```python
from build123d import *

# Parameters (mm, degrees)
SKETCH1_W               = 1.5
SKETCH1_H               = 620
BOSS_EXTRUDE1_DEPTH     = 1.5
BOSS_EXTRUDE3_DEPTH     = 1.5
SKETCH5_W               = 1.5
SKETCH5_H               = 1.5
CUT_EXTRUDE1_DEPTH      = 1
CUT_EXTRUDE1_DEPTH_BACK = 621
BOSS_EXTRUDE4_DEPTH     = 620
SKETCH6_R               = 5
CUT_EXTRUDE2_DEPTH      = 1
CUT_EXTRUDE2_DEPTH_BACK = 57.5
SKETCH7_R               = 5
CUT_EXTRUDE3_DEPTH      = 1
CUT_EXTRUDE3_DEPTH_BACK = 57.5


with BuildPart() as part:
    # Sketch1 → Boss-Extrude1 (new body)
    with BuildSketch(Plane(origin=(0, 0, 0), x_dir=(0, 0, -1), z_dir=(1, 0, 0))):
        Polygon((0, 255), (0, -255), (55, -310), (55, 310), align=None)
        with Locations((55.75, 0)):
            Rectangle(SKETCH1_W, SKETCH1_H)
    extrude(amount=BOSS_EXTRUDE1_DEPTH)

    # Sketch2 → Boss-Extrude3 (add)
    with BuildSketch(Plane(origin=(0, 0, -56.5), x_dir=(-1, 0, 0), z_dir=(0, 0, -1))):
        Polygon((55, 255), (55, -255), (0, -310), (0, 310), align=None)
    extrude(amount=-BOSS_EXTRUDE3_DEPTH)

    # Sketch5 → Cut-Extrude1 (cut, two sides)
    with BuildSketch(Plane.XZ.offset(310)) as cut_extrude1_sk:
        with BuildLine():
            ThreePointArc((1.5, -44.5), (-2.014718626, -52.985281374), (-10.5, -56.5))
            Line((-10.5, -56.5), (0, -56.5))
            Line((0, -56.5), (0, -55))
            Line((0, -55), (1.5, -55))
            Line((1.5, -55), (1.5, -44.5))
        make_face()
        with Locations((0.75, -55.75)):
            Rectangle(SKETCH5_W, SKETCH5_H)
    extrude(amount=CUT_EXTRUDE1_DEPTH, mode=Mode.SUBTRACT)
    extrude(cut_extrude1_sk.sketch, amount=-CUT_EXTRUDE1_DEPTH_BACK, mode=Mode.SUBTRACT)

    # Sketch5<3> → Boss-Extrude4 (add)
    with BuildSketch(Plane.XZ.offset(310)):
        with BuildLine():
            Line((-10.5, -55), (-10.5, -56.5))
            ThreePointArc((-10.5, -56.5), (-2.014718626, -52.985281374), (1.5, -44.5))
            Line((1.5, -44.5), (0, -44.5))
            ThreePointArc((0, -44.5), (-3.075378798, -51.924621202), (-10.5, -55))
        make_face()
    extrude(amount=-BOSS_EXTRUDE4_DEPTH)

    # Sketch6 → Cut-Extrude2 (cut, two sides)
    with BuildSketch(Plane(origin=(1.5, 0, 0), x_dir=(0, 0, -1), z_dir=(1, 0, 0))) as cut_extrude2_sk:
        with Locations((24.5, 0)):
            Circle(SKETCH6_R)
    extrude(amount=CUT_EXTRUDE2_DEPTH, mode=Mode.SUBTRACT)
    extrude(cut_extrude2_sk.sketch, amount=-CUT_EXTRUDE2_DEPTH_BACK, mode=Mode.SUBTRACT)

    # Sketch7 → Cut-Extrude3 (cut, two sides)
    with BuildSketch(Plane(origin=(0, 0, -56.5), x_dir=(-1, 0, 0), z_dir=(0, 0, -1))) as cut_extrude3_sk:
        with Locations((30.5, 0)):
            Circle(SKETCH7_R)
    extrude(amount=CUT_EXTRUDE3_DEPTH, mode=Mode.SUBTRACT)
    extrude(cut_extrude3_sk.sketch, amount=-CUT_EXTRUDE3_DEPTH_BACK, mode=Mode.SUBTRACT)


solid = part.part
```
Geometry check sheet. Reference: the model listing, model coordinates, mm. A direction names the side the tool comes from. Give positions to 0.01 mm unless a question says otherwise; leave off trailing zeros. Order: outer loops, then holes, each group sorted by start corner. A loop starts at its lowest first (then second) coordinate and runs counter-clockwise, first axis right, second up.
1. Thickness scan on L1, parallel to Y at x = 0.95, z = -24.5; L2, parallel to X at y = 90.5, z = -23; L3, parallel to Z at x = -31.5, y = 165. Record the ranges inside material, lowest first.
2. Section check C-C, the plane z = -13. Enter the section's corners in (x, y), and give its area (3 significant figures).
3. Section check A-A, the plane y = -206.5. Enter the section's corners in (x, z), and give its area (3 significant figures).
4. Release check for a two-part mould opening along Y. For faces 1 (the face through (0.76, 0.22, -19.505)), 2 (the face through (1, -277, -22)), 3 (the face through (-38, 4, -55)) record: pulls with the +Y half, pulls with the -Y half, needs draft (parallel to the pull), parting line crosses it, or undercut.
5. Access from +Z, -Z, +X, -X, +Y, -Y to the whole of each face (thin tool, end or side, straight path). Record for faces 4 (the face through (0, 4, -17)), 5 (the face through (-2.11, -4.34, -53.08)).
6. Section check B-B, the plane x = -19. Enter the section's corners in (y, z), and give its area (3 significant figures).
7. Gauge pin test, flat ends, axial feed: pin 1 Ø2 at (x, y) = (-6.5, 150) entering from -Z; pin 2 Ø8 at (x, y) = (-28.5, 149) entering from +Z; pin 3 Ø1.6 at (x, y) = (0.5, -302.5) entering from +Z. Record the tip position at first contact, or that the pin passes through.
Values follow:
1. L1: y = -279.5 to -5, 5 to 279.5
1. L2: x = 0 to 1.5
1. L3: z = -56.5 to -55
2. outline: (0, -268) - (1.5, -268) - (1.5, 268) - (0, 268) - close
2. area: 804 mm2
3. outline: (-55, -56.5) - (-10.5, -56.5) arc R12 ccw to (1.5, -44.5) - (1.5, 0) - (0, 0) - (0, -44.5) arc R10.5 cw to (-10.5, -55) - (-55, -55) - close
3. area: 160 mm2
4. face 1: undercut
4. face 2: pulls with the -Y half
4. face 3: needs draft
5. face 4: +Z, -X, +Y, -Y
5. face 5: -Z, +X, +Y, -Y
6. outline: (-291, -56.5) - (291, -56.5) - (291, -55) - (-291, -55) - close
6. area: 873 mm2
7. pin 1: stops at z = -56.12
7. pin 2: stops at z = -55
7. pin 3: stops at z = -44.5
